Source: three-view drawing plus pictorial views. Frame: mm from the lowest corner of the part. A direction names the side the tool comes from. Coordinates: 2 decimals unless noted, no trailing zeros. Write each loop counter-clockwise with the first axis right and the second up, starting at its lowest first coordinate (ties: lowest second). Pieces come first, ordered by that corner, then holes. Notation, with made-up numbers: (21.5, 48) - (52.5, 48) arc R15 cw to (52.5, 65) - close; hole circle Ø10 at (67, 11). An arc over 180 degrees is marked (long way). Put each result on its own line as item: value.
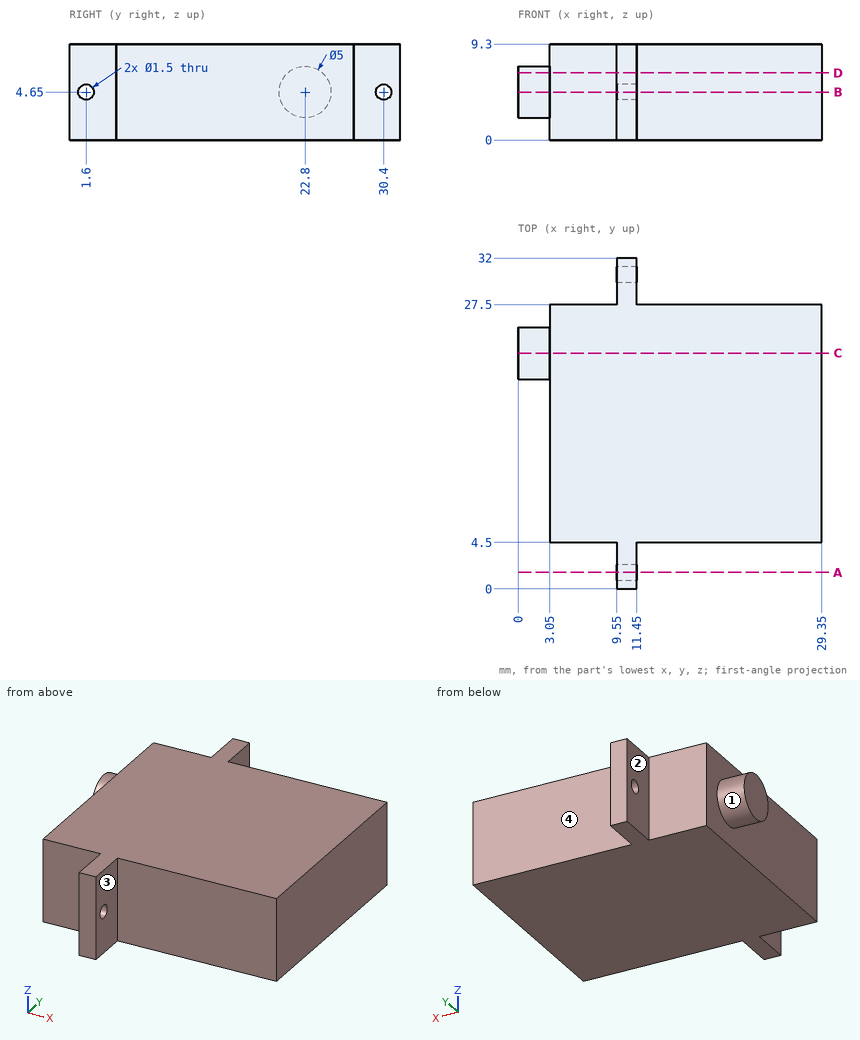
1. Section query C-C (y = 22.8). Return loops of the section in (x, z), then the cut area to 3 significant figures.
Answer below:
outline: (0, 2.15) - (3.05, 2.15) - (3.05, 0) - (29.35, 0) - (29.35, 9.3) - (3.05, 9.3) - (3.05, 7.15) - (0, 7.15) - close
area: 260 mm²
2. Ray query, probe 1 along Z at (x, y) = (10.25, 1.6); probe 2 along Y at (x, z) = (22.25, 7.5); probe 3 along X at (y, z) = (7, 8.75). Return the intervals inside material, ascending. Write a range as from..to.
Answer below:
probe 1: z = 0..3.9, 5.4..9.3
probe 2: y = 4.5..27.5
probe 3: x = 3.05..29.35
3. Section query B-B (z = 4.65). Return loops of the section in (x, y), then the cut area to 3 significant figures.
Answer below:
outline: (0, 20.3) - (3.05, 20.3) - (3.05, 4.5) - (9.55, 4.5) - (9.55, 2.35) - (11.45, 2.35) - (11.45, 4.5) - (29.35, 4.5) - (29.35, 27.5) - (11.45, 27.5) - (11.45, 29.65) - (9.55, 29.65) - (9.55, 27.5) - (3.05, 27.5) - (3.05, 25.3) - (0, 25.3) - close; (9.55, 0) - (11.45, 0) - (11.45, 0.85) - (9.55, 0.85) - close; (9.55, 31.15) - (11.45, 31.15) - (11.45, 32) - (9.55, 32) - close
area: 632 mm²
4. Section query D-D (z = 6.5). Return loops of the section in (x, y), then the cut area to 3 significant figures.
Answer below:
outline: (0, 21.12) - (3.05, 21.12) - (3.05, 4.5) - (9.55, 4.5) - (9.55, 0) - (11.45, 0) - (11.45, 4.5) - (29.35, 4.5) - (29.35, 27.5) - (11.45, 27.5) - (11.45, 32) - (9.55, 32) - (9.55, 27.5) - (3.05, 27.5) - (3.05, 24.48) - (0, 24.48) - close
area: 632 mm²
5. Pin query (flat end, axial travel): pin 1 Ø1 at (y, z) = (11.5, 6.5) entering from -X; pin 2 Ø3 at (x, z) = (18, 3) entering from -Y; pin 3 Ø3 at (x, z) = (7.5, 6.5) entering from +Y; pin 4 Ø2 at (y, z) = (25.5, 5) entering from -X. Return the tip coordinate at first contact, or that it passes through.
Answer below:
pin 1: stops at x = 3.05
pin 2: stops at y = 4.5
pin 3: stops at y = 27.5
pin 4: stops at x = 0
6. Set-up query: the marked faces 1, 2, 3 and 4. Return all of +Z, -Z, +X, -X, +Y, -Y with unobstructed straight access to the full face (end or side cutting, diameter ignored); none if empty.
Answer below:
face 1: -X
face 2: +Z, -Z, -X, +Y
face 3: +Z, -Z, +X, -Y
face 4: +Z, -Z, +X, +Y
7. Section query A-A (y = 1.6). Return loops of the section in (x, z), then the cut area to 3 significant figures.
Answer below:
outline: (9.55, 0) - (11.45, 0) - (11.45, 3.9) - (9.55, 3.9) - close; (9.55, 5.4) - (11.45, 5.4) - (11.45, 9.3) - (9.55, 9.3) - close
area: 14.8 mm²
